Input: part model. Units: mm. Frame: model coordinates. Face numbers are marked on the shaded views. A direction names the side the tool comes from. Coordinates: 2 decimals unless noted, no trailing zeros. Write each loop counter-clockwise with the first axis right and the second up, starting at its lowest first coordinate (ties: lowest second). Pieces come first, ordered by that corner, then holes. Notation, with made-up numbers: (83.5, 4) -> (136.5, 4) arc R12 ccw to (136.5, 12) -> close; hole circle Ø6 at (42, 74). An arc over 180 degrees is marked (long way). Use one line per item in the form item = value. Start each with the question number.
(1) Cut plane B-B on x = 13. Return the cut outline in (y, z), plus the area to 3 significant figures.
(2) Set-up query: the marked faces 1, 2 and 3. Return all of +Z, -Z, +X, -X, +Y, -Y with unobstructed straight access to the full face (end or side cutting, diameter ignored); none if empty.
(3) Cut plane A-A on z = 0. Return the cut outline in (x, y).
(4) Cut plane C-C on y = 4.5. Return the cut outline in (x, z), plus the area to 3 significant figures.
(5) Ray query, line 1 along Y through (x, z) = (-31, 2); line 2 along X through (y, z) = (-3, -5.5); line 3 along Y through (x, z) = (7, 9). Return the intervals inside material, ascending.
(6) Pull-direction query (Z, two-part tool) for the marked faces 4, 5 and 6; classes: released by +Z, released by -Z, zero draft, split by the parting line, or undercut.
(7) Cut plane D-D on z = 13. Return the cut outline in (x, y).
(8) First-contact query: pin 1 (5 mm diameter, centred on x = -10.5, z = 8.5, fed in from -Y); pin 2 (1.8 mm diameter, centred on y = 3.5, z = -14, fed in from -X); pin 3 (1.8 mm diameter, centred on y = -2.5, z = -9, fed in from -X). Flat tips, straight axial feed; report the tip coordinate or a pass-through.
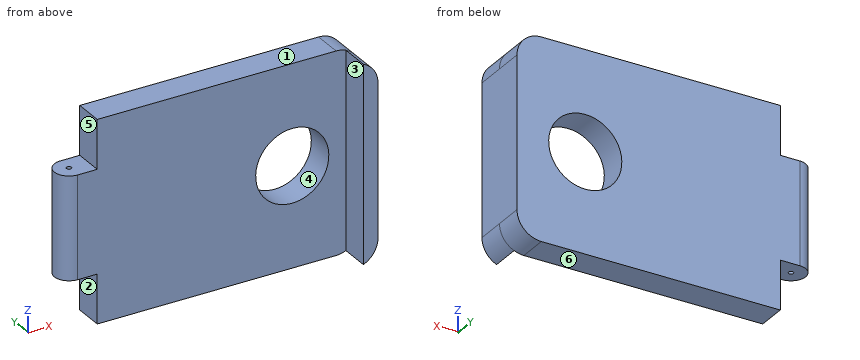
```python
from build123d import *

# Parameters (mm, degrees)
EXTRUDE_1_DEPTH     = 6
FILLET_1_RADIUS     = 3
FILLET_1_LENGTH     = 21
SKETCH_2_R          = 7.5
CUT_EXTRUDE_1_DEPTH = 6
FILLET_2_R          = 5
FILLET_3_R          = 5
EXTRUDE_2_DEPTH     = 6
SKETCH_4_R          = 0.5
CUT_EXTRUDE_2_DEPTH = 21


with BuildPart() as part:
    # Эскиз1 → Бобышка-Вытянуть1 (new body)
    with BuildSketch(Plane(origin=(0, 0, 0), x_dir=(1, 0, 0), z_dir=(0, 1, 0))):
        Polygon((-27, -20.5), (27, -20.5), (27, 20.5), (-27, 20.5), (-27, 10.5), (-34, 10.5), (-34, -10.5), (-27, -10.5), align=None)
    extrude(amount=EXTRUDE_1_DEPTH)

    # Скругление1: full round fillet: the end face becomes a half cylinder, R = half its width
    fillet_1_face = Plane((-34, 3, 0), x_dir=(0, 0, -1), z_dir=(-1, 0, 0))  # on the end face: x along it, z out of the body
    fillet_1_slab = fillet_1_face.offset(-FILLET_1_RADIUS / 2) * Box(FILLET_1_LENGTH, 2 * FILLET_1_RADIUS, FILLET_1_RADIUS, mode=Mode.PRIVATE)  # the body's end, R deep
    fillet_1_round = Plane((-31, 3, 0), x_dir=(-1, 0, 0), z_dir=(0, 0, -1)) * Cylinder(FILLET_1_RADIUS, FILLET_1_LENGTH, mode=Mode.PRIVATE)  # its axis R under the face
    add(fillet_1_slab - fillet_1_round, mode=Mode.SUBTRACT)

    # Эскиз2 → Вырез-Вытянуть1 (cut)
    with BuildSketch(Plane(origin=(0, 6, 0), x_dir=(1, 0, 0), z_dir=(0, 1, 0))):
        with Locations(Location((13, 0, 0), (0, 0, 270))):
            Circle(SKETCH_2_R)
    extrude(amount=-CUT_EXTRUDE_1_DEPTH, mode=Mode.SUBTRACT)

    # Скругление2
    fillet_2_edges = [part.edges().sort_by_distance(p)[0] for p in [
        (27, 3, -20.5),
    ]]
    fillet(fillet_2_edges, radius=FILLET_2_R)

    # Скругление3
    fillet_3_edges = [part.edges().sort_by_distance(p)[0] for p in [
        (27, 3, 20.5),
    ]]
    fillet(fillet_3_edges, radius=FILLET_3_R)

    # Эскиз3 → Бобышка-Вытянуть2 (add)
    with BuildSketch(Plane.XZ):
        with BuildLine():
            Line((24, 15.5), (24, -20.082575695))
            ThreePointArc((24, -20.082575695), (26.183300133, -18.238612788), (27, -15.5))
            Line((27, -15.5), (27, 15.5))
            ThreePointArc((27, 15.5), (26.183300133, 18.238612788), (24, 20.082575695))
            Line((24, 20.082575695), (24, 15.5))
        make_face()
    extrude(amount=EXTRUDE_2_DEPTH)

    # Эскиз4 → Вырез-Вытянуть2 (cut)
    with BuildSketch(Plane.XY.offset(10.5)):
        with Locations((-31, 3)):
            Circle(SKETCH_4_R)
    extrude(amount=-CUT_EXTRUDE_2_DEPTH, mode=Mode.SUBTRACT)


solid = part.part
```
Values:
q1.outline = (0, -20.5) -> (6, -20.5) -> (6, -7.5) -> (0, -7.5) -> close; (0, 7.5) -> (6, 7.5) -> (6, 20.5) -> (0, 20.5) -> close
q1.area = 156 mm2
q2.face_1 = +Z, +X, -X, +Y, -Y
q2.face_2 = -Z, -X, +Y, -Y
q2.face_3 = +Z, -Z, -X, -Y
q3.outline = (-31, 0) -> (5.5, 0) -> (5.5, 6) -> (-31, 6) arc R3 ccw to start; (20.5, 0) -> (24, 0) -> (24, -6) -> (27, -6) -> (27, 6) -> (20.5, 6) -> close; hole circle Ø1 at (-31, 3)
q4.outline = (-33.6, -10.5) -> (-27, -10.5) -> (-27, -20.5) -> (22, -20.5) arc R5 ccw to (27, -15.5) -> (27, 15.5) arc R5 ccw to (22, 20.5) -> (-27, 20.5) -> (-27, 10.5) -> (-33.6, 10.5) -> close; hole circle Ø15 at (13, 0)
q4.area = 2,170 mm2
q5.line_1 = 0 to 2.5, 3.5 to 6
q5.line_2 = 24 to 27
q5.line_3 = 0 to 6
q6.face_4 = undercut
q6.face_5 = zero draft
q6.face_6 = released by -Z
q7.outline = (-27, 0) -> (24, 0) -> (24, -6) -> (27, -6) -> (27, 6) -> (-27, 6) -> close
q8.pin_1 = 0
q8.pin_2 = -27
q8.pin_3 = 24
